from build123d import *

# Parameters (mm, degrees)
SKETCH_1_W          = 130
SKETCH_1_H          = 82
EXTRUDE_1_DEPTH     = 8
SKETCH_2_R          = 2.1
CUT_EXTRUDE_1_DEPTH = 142.58762947
SKETCH_3_W          = 110
SKETCH_3_H          = 82
EXTRUDE_2_DEPTH     = 8
SKETCH_4_W          = 110
SKETCH_4_H          = 2
CUT_EXTRUDE_2_DEPTH = 125.141148579
SKETCH_7_W          = 6
SKETCH_7_H          = 8
CUT_EXTRUDE_3_DEPTH = 10


with BuildPart() as part:
    # 草圖1 → 填料-伸長1 (new body)
    with BuildSketch(Plane.XY):
        with Locations((27.860243218, 14.525280899)):
            Rectangle(SKETCH_1_W, SKETCH_1_H)
    extrude(amount=EXTRUDE_1_DEPTH)

    # 草圖2 → 除料-伸長1 (cut, through all)
    with BuildSketch(Plane.ZY.offset(37.139756782)):
        with Locations((4, -22.474719101)):
            Circle(SKETCH_2_R)
        with Locations((4, -6.474719101)):
            Circle(SKETCH_2_R)
        with Locations((4, 9.525280899)):
            Circle(SKETCH_2_R)
        with Locations((4, 19.525280899)):
            Circle(SKETCH_2_R)
        with Locations((4, 35.525280899)):
            Circle(SKETCH_2_R)
        with Locations((4, 51.525280899)):
            Circle(SKETCH_2_R)
    extrude(amount=-CUT_EXTRUDE_1_DEPTH, mode=Mode.SUBTRACT)

    # 草圖3 → 填料-伸長2 (add)
    with BuildSketch(Plane(origin=(0, 0, 0), x_dir=(-1, 0, 0), z_dir=(0, 0, -1))):
        with Locations((-27.860243218, 14.525280899)):
            Rectangle(SKETCH_3_W, SKETCH_3_H)
    extrude(amount=-EXTRUDE_2_DEPTH)

    # 草圖4 → 除料-伸長2 (cut, through all)
    with BuildSketch(Plane.XZ.offset(26.474719101)):
        with Locations((27.860243218, 7)):
            Rectangle(SKETCH_4_W, SKETCH_4_H)
        with Locations((27.860243218, 1)):
            Rectangle(SKETCH_4_W, SKETCH_4_H)
    extrude(amount=-CUT_EXTRUDE_2_DEPTH, mode=Mode.SUBTRACT)

    # 草圖7 → 除料-伸長3 (cut)
    with BuildSketch(Plane.XY.offset(8)):
        with Locations((-26.139756782, 51.525280899)):
            Rectangle(SKETCH_7_W, SKETCH_7_H)
        with Locations((81.860243218, 51.525280899)):
            Rectangle(SKETCH_7_W, SKETCH_7_H)
        with Locations((-26.139756782, 35.525280899)):
            Rectangle(SKETCH_7_W, SKETCH_7_H)
        with Locations((81.860243218, 35.525280899)):
            Rectangle(SKETCH_7_W, SKETCH_7_H)
        with Locations((-26.139756782, 19.525280899)):
            Rectangle(SKETCH_7_W, SKETCH_7_H)
        with Locations((81.860243218, 19.525280899)):
            Rectangle(SKETCH_7_W, SKETCH_7_H)
        with Locations((-26.139756782, 9.525280899)):
            Rectangle(SKETCH_7_W, SKETCH_7_H)
        with Locations((81.860243218, 9.525280899)):
            Rectangle(SKETCH_7_W, SKETCH_7_H)
        with Locations((-26.139756782, -6.474719101)):
            Rectangle(SKETCH_7_W, SKETCH_7_H)
        with Locations((81.860243218, -6.474719101)):
            Rectangle(SKETCH_7_W, SKETCH_7_H)
        with Locations((-26.139756782, -22.474719101)):
            Rectangle(SKETCH_7_W, SKETCH_7_H)
        with Locations((81.860243218, -22.474719101)):
            Rectangle(SKETCH_7_W, SKETCH_7_H)
    extrude(amount=-CUT_EXTRUDE_3_DEPTH, mode=Mode.SUBTRACT)


solid = part.part
Read the model definition and answer for the solid it produces. Units are mm, in the model's axes. A direction names the side the tool comes from. Round coordinates to 2 decimals unless told otherwise and drop trailing zeros. Loops run counter-clockwise (first coordinate to the right, second up) from the corner with the lowest first, then second, coordinate; pieces in that order, holes last. Notation, with made-up numbers: (66.25, -19.75) - (107.25, -19.75) arc R20 cw to (107.25, 11.25) - close; hole circle Ø9 at (4.25, 23.5). An arc over 180 degrees is marked (long way). One line per question, with ' | ' between items. Start each with the question number.
Q1. For faces 1 (the flat face through (82, 39.525, 4)), 2 (the cylindrical face through (88.804, 17.662, 4.969)), 3 (the cylindrical face through (-33.196, 49.475, 3.545)), determine the directions among +Z, -Z, +X, -X, +Y, -Y from which every point of the face is accessible in a straight line to the end or side of a thin tool.
Q2. Flat-ended cylindrical pins translate along their axes: pin 1 (1.8 mm diameter, centred on x = 82.5, z = 3, fed in from +Y); pin 2 (3.5 mm diameter, centred on y = -22.47, z = 4, fed in from -X); pin 3 (1.8 mm diameter, centred on x = -26.5, z = 3.5, fed in from -Y). Find the tip coordinate at first contact, or state that the pin passes through.
Q3. Section B-B on y = 41 is taken. Give the vertices of the cut face in (x, z).
Q4. Section C-C on x = 39 is taken. Give the vertices of the cut face in (y, z), plus the area to 3 significant figures.
Q5. Find the intervals of material crossed by L1, parallel to Y at x = -26.5, z = 3.5; L2, parallel to X at y = 8, z = 5.75; L3, parallel to X at y = 0, z = 7.5, in increasing order.
Q6. Section A-A on z = 4 is taken. Count the separate pieces of the cut face and the enclosed holes in it, plus the area to 3 significant figures.
Q7. For a pull along X with two mould halves and no side action, classify faces 4 (the flat face through (-32, 15, 8)), 5 (the flat face through (84.86, 34, 2)), 6 (the flat face through (-37.14, 14, 4)) as +X half, -X half, draft (parallel to the pull), parting line (faces both ways), or undercut.
Established:
1) face 1: +Z, -Z | face 2: +X | face 3: -X
2) pin 1: y = 47.53 | pin 2: x = -23.14 | pin 3: y = -18.47
3) outline: (-37.14, 0) - (-27.14, 0) - (-27.14, 2) - (82.86, 2) - (82.86, 0) - (92.86, 0) - (92.86, 8) - (82.86, 8) - (82.86, 6) - (-27.14, 6) - (-27.14, 8) - (-37.14, 8) - close
4) outline: (-26.47, 2) - (55.53, 2) - (55.53, 6) - (-26.47, 6) - close | area: 328 mm²
5) L1: -18.47 to -10.47, -2.47 to 5.53, 13.53 to 15.53, 23.53 to 31.53, 39.53 to 47.53 | L2: -37.14 to -29.14, -23.14 to 78.86, 84.86 to 92.86 | L3: -37.14 to -27.14, 82.86 to 92.86
6) separate pieces: 5 | enclosed holes: 0 | area: 9,680 mm²
7) face 4: draft | face 5: undercut | face 6: -X half
